from build123d import *

# Parameters (mm, degrees)
BOSS_EXTRUDE1_DEPTH = 5
CUT_EXTRUDE1_START  = -2
CUT_EXTRUDE1_DEPTH  = 2
CUT_EXTRUDE2_DEPTH  = 52.23475383
SKETCH4_R           = 3
CUT_EXTRUDE3_DEPTH  = 2
SKETCH5_W           = 17.5
SKETCH5_H           = 12
SKETCH5_W_2         = 5.5
SKETCH5_R           = 1
CUT_EXTRUDE4_DEPTH  = 52.23475383
BOSS_EXTRUDE2_START = 6
SKETCH6_R           = 1
SKETCH6_W           = 23
SKETCH6_H           = 12
BOSS_EXTRUDE2_DEPTH = 6
FILLET1_R           = 3
FILLET2_R           = 3
SKETCH7_R           = 1.5
CUT_EXTRUDE5_DEPTH  = 4
SKETCH8_R           = 1.75
CUT_EXTRUDE6_DEPTH  = 10


with BuildPart() as part:
    # Sketch1 → Boss-Extrude1 (new body)
    with BuildSketch(Plane(origin=(0, 0, 0), x_dir=(1, 0, 0), z_dir=(0, 1, 0))):
        with BuildLine():
            Line((-40, 10), (40, 10))
            ThreePointArc((40, 10), (50, 0), (40, -10))
            Line((40, -10), (-40, -10))
            ThreePointArc((-40, -10), (-50, 0), (-40, 10))
        make_face()
    extrude(amount=BOSS_EXTRUDE1_DEPTH)

    # Sketch2 → Cut-Extrude1 (cut)
    with BuildSketch(Plane(origin=(0, 5, 0), x_dir=(1, 0, 0), z_dir=(0, 1, 0)).offset(CUT_EXTRUDE1_START)):
        with BuildLine():
            Line((-39.171140726, 3.913181864), (-40, 4))
            Line((-40, 4), (-40.854873646, 3.907581227))
            Line((-40.854873646, 3.907581227), (-49.549514718, 2.96762003))
            ThreePointArc((-49.549514718, 2.96762003), (-50, 0), (-49.549514718, -2.96762003))
            Line((-49.549514718, -2.96762003), (-40.854873646, -3.907581227))
            Line((-40.854873646, -3.907581227), (-40, -4))
            Line((-40, -4), (-39.171140726, -3.913181864))
            Line((-39.171140726, -3.913181864), (-20.905849501, -2))
            ThreePointArc((-20.905849501, -2), (-18.905849501, 0), (-20.905849501, 2))
            Line((-20.905849501, 2), (-39.171140726, 3.913181864))
        make_face()
    extrude(amount=CUT_EXTRUDE1_DEPTH, mode=Mode.SUBTRACT)

    # Sketch3 → Cut-Extrude2 (cut, through all)
    with BuildSketch(Plane(origin=(0, 5, 0), x_dir=(1, 0, 0), z_dir=(0, 1, 0))):
        with BuildLine():
            ThreePointArc((-39, 0), (-39.292893219, 0.707106781), (-40, 1))
            Line((-40, 1), (-40, -1))
            ThreePointArc((-40, -1), (-39.292893219, -0.707106781), (-39, 0))
        make_face()
        with BuildLine():
            Line((-40, -1), (-40, 1))
            ThreePointArc((-40, 1), (-41, 0), (-40, -1))
        make_face()
    extrude(amount=-CUT_EXTRUDE2_DEPTH, mode=Mode.SUBTRACT)

    # Sketch4 → Cut-Extrude3 (cut)
    with BuildSketch(Plane.XZ):
        with Locations(Location((-40, 0, 0), (0, 0, 270))):
            Circle(SKETCH4_R)
    extrude(amount=-CUT_EXTRUDE3_DEPTH, mode=Mode.SUBTRACT)

    # Sketch5 → Cut-Extrude4 (cut, through all)
    with BuildSketch(Plane(origin=(0, 5, 0), x_dir=(1, 0, 0), z_dir=(0, 1, 0))):
        with Locations((31.25, 0)):
            Rectangle(SKETCH5_W, SKETCH5_H)
        with Locations((42.75, 0)):
            Rectangle(SKETCH5_W_2, SKETCH5_H)
        with Locations(Location((47.5, 0, 0), (0, 0, 270))):
            Circle(SKETCH5_R)
        with Locations(Location((20.5, 0, 0), (0, 0, 270))):
            Circle(SKETCH5_R)
    extrude(amount=-CUT_EXTRUDE4_DEPTH, mode=Mode.SUBTRACT)

    # Sketch6 → Boss-Extrude2 (add)
    with BuildSketch(Plane(origin=(0, 5, 0), x_dir=(1, 0, 0), z_dir=(0, 1, 0)).offset(BOSS_EXTRUDE2_START)):
        with BuildLine():
            Line((15.501327646, 10), (15.501327646, -10))
            Line((15.501327646, -10), (40, -10))
            ThreePointArc((40, -10), (50, 0), (40, 10))
            Line((40, 10), (15.501327646, 10))
        make_face()
        with Locations(Location((20.5, 0, 0), (0, 0, 270))):
            Circle(SKETCH6_R, mode=Mode.SUBTRACT)
        with Locations(Location((47.5, 0, 0), (0, 0, 270))):
            Circle(SKETCH6_R, mode=Mode.SUBTRACT)
        with Locations((34, 0)):
            Rectangle(SKETCH6_W, SKETCH6_H, mode=Mode.SUBTRACT)
    extrude(amount=-BOSS_EXTRUDE2_DEPTH)

    # Fillet1
    fillet1_edges = [part.edges().sort_by_distance(p)[0] for p in [
        (15.501327646, 11, 0),
    ]]
    fillet(fillet1_edges, radius=FILLET1_R)

    # Fillet2
    fillet2_edges = [part.edges().sort_by_distance(p)[0] for p in [
        (15.501327646, 5, 0),
    ]]
    fillet(fillet2_edges, radius=FILLET2_R - 0.0001)  # a hair under: the kernel refuses the full size

    # Sketch7 → Cut-Extrude5 (cut)
    with BuildSketch(Plane.XZ):
        with Locations(Location((20.5, 0, 0), (0, 0, 270))):
            Circle(SKETCH7_R)
        with Locations(Location((47.5, 0, 0), (0, 0, 270))):
            Circle(SKETCH7_R)
    extrude(amount=-CUT_EXTRUDE5_DEPTH, mode=Mode.SUBTRACT)

    # Sketch8 → Cut-Extrude6 (cut)
    with BuildSketch(Plane(origin=(0, 0, -10), x_dir=(-1, 0, 0), z_dir=(0, 0, -1))):
        with Locations((0, 2.5)):
            Circle(SKETCH8_R)
    extrude(amount=-CUT_EXTRUDE6_DEPTH, mode=Mode.SUBTRACT)


solid = part.part
Design review of the part built by this model. Coordinates are the model's own, in mm. A direction names the side the tool comes from. Round coordinates to 2 decimals unless told otherwise and drop trailing zeros. Write each loop counter-clockwise with the first axis right and the second up, starting at its lowest first coordinate (ties: lowest second). Pieces come first, ordered by that corner, then holes. Notation, with made-up numbers: (-9.75, -6) - (34.25, -6) arc R30 cw to (34.25, 21) - close; hole circle Ø2 at (3, 62). An arc over 180 degrees is marked (long way). Return JSON: item names as keys, results as strings. Group by question number.
Item 1: We need section A-A on x = 39. Write out the cut boundary in (y, z).
Item 2: Insertion check: P1, Ø0.9, axis at x = 20, z = 0.5, coming from the -Y side; P2, Ø10, axis at x = -34, z = 3.5, coming from the +Y side; P3, Ø6, axis at y = 6.5, z = 3.5, coming from the -X side. Each pin has a flat end and moves straight along its axis. Give the tip position at first contact, or say it passes through.
Item 3: We need section C-C on y = 6.75. Write out the cut boundary in (x, z), and give its area (3 significant figures).
Item 4: Machinability: for faces 1 (the face through (-0.81, 0.95, -5.07)), 2 (the face through (34, 6, 6)), 3 (the face through (46, 2, 0)), which of the approach directions +Z, -Z, +X, -X, +Y, -Y give a long, thin tool a straight path to every point of the face, cutting with its end or side? Answer none if there is none.
Item 5: The part is to be moulded in two halves that separate along Z. For faces 4 (the face through (14.646, 5.902, 0.14)), 5 (the face through (22.5, 6, 0)), 6 (the face through (0, 3, 0)), say which applies: pulls with the +Z half, pulls with the -Z half, needs draft (parallel to the pull), parting line crosses it, or undercut.
Item 6: We need section B-B on x = 0. Write out the cut boundary in (y, z), and give its area (3 significant figures).
Item 7: For probe 1 along Z at (x, y) = (32, 3); probe 2 along Y at (x, z) = (0, -5.5); probe 3 along Y at (x, z) = (-14, 4.75), list the stretches that pass through material, from the lowest coordinate up. Write a range as [from, to].
Model answer:
{
 "1": {"outline": "(0, -10) - (11, -10) - (11, -6) - (0, -6) - close; (0, 6) - (11, 6) - (11, 10) - (0, 10) - close"},
 "2": {"P1": "stops at y = 4", "P2": "stops at y = 5", "P3": "stops at x = -49.55"},
 "3": {"outline": "(15.23, -10) - (40, -10) arc R10 ccw to (40, 10) - (15.23, 10) - close; hole circle Ø2 at (20.5, 0); hole (22.5, -6) - (45.5, -6) - (45.5, 6) - (22.5, 6) - close; hole circle Ø2 at (47.5, 0)", "area": "370 mm²"},
 "4": {"face 1": "-Z", "face 2": "+Y, -Y", "face 3": "-Y"},
 "5": {"face 4": "needs draft", "face 5": "undercut", "face 6": "pulls with the -Z half"},
 "6": {"outline": "(0, -10) - (0.75, -10) - (0.75, 0) - (4.25, 0) - (4.25, -10) - (5, -10) - (5, 10) - (0, 10) - close", "area": "65.0 mm²"},
 "7": {"probe 1": "z = [-10, -6], [6, 10]", "probe 2": "y = [0, 0.75], [4.25, 5]", "probe 3": "y = [0, 5]"}
}
